Read the model definition and answer for the solid it produces. Units are mm, in the model's axes. Give positions to 0.01 mm unless a question says otherwise; leave off trailing zeros. Write each loop counter-clockwise with the first axis right and the second up, starting at its lowest first coordinate (ties: lowest second). Pieces come first, ordered by that corner, then holes.
```python
from build123d import *

# Parameters (mm, degrees)
PAD_DEPTH       = 12
SKETCH004_R     = 25
POCKET001_DEPTH = 20
SKETCH005_R     = 1.5
POCKET_DEPTH    = 12.001
SKETCH006_W     = 310
SKETCH006_H     = 22
POCKET002_DEPTH = 1


with BuildPart() as part:
    # Sketch (on Part) → Pad (new body)
    with BuildSketch(Plane.XY):
        Polygon((0, 413.879036), (0, 495), (450, 495), (450, 0), (0, 0), align=None)
    extrude(amount=-PAD_DEPTH)

    # Sketch004 → Pocket001 (cut)
    with BuildSketch(Plane.XY):
        with Locations((393.308105, 437.5)):
            Circle(SKETCH004_R)
        with Locations((393.308105, 57.5)):
            Circle(SKETCH004_R)
        with Locations((310, 107.5)):
            Circle(SKETCH004_R)
        with Locations((310, 387.5)):
            Circle(SKETCH004_R)
    extrude(amount=-POCKET001_DEPTH, mode=Mode.SUBTRACT)

    # Sketch005 → Pocket (cut, through all)
    with BuildSketch(Plane.XY):
        with Locations((30, 397.5)):
            Circle(SKETCH005_R)
        with Locations((30, 97.5)):
            Circle(SKETCH005_R)
    extrude(amount=-POCKET_DEPTH, mode=Mode.SUBTRACT)

    # Sketch006 → Pocket002 (cut)
    with BuildSketch(Plane.XY):
        with Locations((275, 11)):
            Rectangle(SKETCH006_W, SKETCH006_H)
        with Locations((275, 484)):
            Rectangle(SKETCH006_W, SKETCH006_H)
    extrude(amount=-POCKET002_DEPTH, mode=Mode.SUBTRACT)


solid = part.part
```
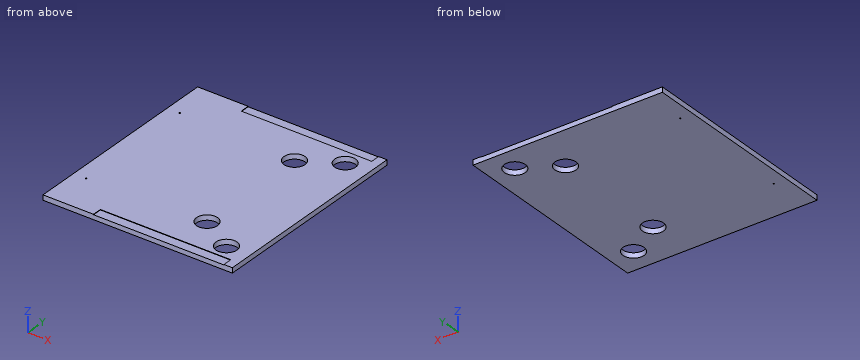
Item 1: Section A-A (x = 310) is taken. Write down the section's boundary in (y, z).
Result set:
outline: (0, -12) - (82.5, -12) - (82.5, 0) - (22, 0) - (22, -1) - (0, -1) - close; (132.5, -12) - (362.5, -12) - (362.5, 0) - (132.5, 0) - close; (412.5, -12) - (495, -12) - (495, -1) - (473, -1) - (473, 0) - (412.5, 0) - close
Item 2: Section B-B (y = 437.5) is taken. Write down the section's boundary in (x, z), and give its area (3 significant figures).
Result set:
outline: (0, -12) - (368.31, -12) - (368.31, 0) - (0, 0) - close; (418.31, -12) - (450, -12) - (450, 0) - (418.31, 0) - close
area: 4,800 mm2
Item 3: Section C-C (z = -7) is taken. Write down the section's boundary in (x, y), and give its area (3 significant figures).
Result set:
outline: (0, 0) - (450, 0) - (450, 495) - (0, 495) - close; hole circle Ø3 at (30, 97.5); hole circle Ø3 at (30, 397.5); hole circle Ø50 at (310, 107.5); hole circle Ø50 at (310, 387.5); hole circle Ø50 at (393.31, 57.5); hole circle Ø50 at (393.31, 437.5)
area: 215,000 mm2
Item 4: Each of these flat-tipped pins is pushed along its axis until it touches: pin 1 Ø17.5 at (x, y) = (297.5, 488) entering from +Z; pin 2 Ø0.5 at (x, z) = (335, -0.5) entering from -Y. Where does it stop, or does it pass through?
Result set:
pin 1: stops at z = -1
pin 2: stops at y = 22
Item 5: Find the intervals of material crossed by line 1 along Y through (x, z) = (30, -7); line 2 along Y through (x, z) = (310, -2.5); line 3 along X through (y, z) = (389.5, -8.5), in increasing order.
Result set:
line 1: y = 0 to 96, 99 to 396, 399 to 495
line 2: y = 0 to 82.5, 132.5 to 362.5, 412.5 to 495
line 3: x = 0 to 285.08, 334.92 to 450
